```python
from build123d import *

# Parameters (mm, degrees)
SKETCH1_R           = 22.5
SKETCH1_R_2         = 15
SKETCH1_R_3         = 2
BOSS_EXTRUDE1_DEPTH = 5
SKETCH4_R           = 15
SKETCH4_R_2         = 10
SKETCH5_W           = 40
SKETCH5_H           = 40
SKETCH5_R           = 10
SKETCH5_R_2         = 2
BOSS_EXTRUDE2_DEPTH = 5
FILLET1_R           = 4
SKETCH6_R           = 3
BOSS_EXTRUDE3_DEPTH = 7


with BuildPart() as part:
    # Sketch1 → Boss-Extrude1 (new body)
    with BuildSketch(Plane.XY):
        Circle(SKETCH1_R)
        Circle(SKETCH1_R_2, mode=Mode.SUBTRACT)
        with Locations((13.177680547, 13.177680547)):
            Circle(SKETCH1_R_3, mode=Mode.SUBTRACT)
        with Locations((13.177680547, -13.177680547)):
            Circle(SKETCH1_R_3, mode=Mode.SUBTRACT)
        with Locations((-13.177680547, -13.177680547)):
            Circle(SKETCH1_R_3, mode=Mode.SUBTRACT)
        with Locations((-13.177680547, 13.177680547)):
            Circle(SKETCH1_R_3, mode=Mode.SUBTRACT)
    extrude(amount=BOSS_EXTRUDE1_DEPTH)

    # Sweep1: sweep along a path in Sketch3
    with BuildLine(Plane(origin=(0, 0, 0), x_dir=(1, 0, 0), z_dir=(0, 1, 0))) as sweep1_path:
        Line((0, 2.5), (0, -10))
        ThreePointArc((0, -10), (-11.757890636, -42.210884362), (-41.501642855, -59.272486499))
        Line((-41.501642855, -59.272486499), (-53.81976448, -61.397075786))
    # Sketch4 → Sweep1 (sweep)
    with BuildSketch(Plane(origin=(-53.81976448, 0, 61.397075786), x_dir=(0.16996714290024248, 0, 0.98544972998846), z_dir=(-0.98544972998846, 0, 0.16996714290024248))):
        Circle(SKETCH4_R)
        Circle(SKETCH4_R_2, mode=Mode.SUBTRACT)
    sweep(path=sweep1_path.line)

    # Sketch5 → Boss-Extrude2 (add)
    with BuildSketch(Plane(origin=(-62.548620892, 0, 10.788181337), x_dir=(0.16996714290024248, 0, 0.98544972998846), z_dir=(-0.98544972998846, 0, 0.16996714290024248))):
        with Locations((51.356140155, 0)):
            Rectangle(SKETCH5_W, SKETCH5_H)
        with Locations((51.356140155, 0)):
            Circle(SKETCH5_R, mode=Mode.SUBTRACT)
        with Locations((67.356140155, 16)):
            Circle(SKETCH5_R_2, mode=Mode.SUBTRACT)
        with Locations((35.356140155, 16)):
            Circle(SKETCH5_R_2, mode=Mode.SUBTRACT)
        with Locations((35.356140155, -16)):
            Circle(SKETCH5_R_2, mode=Mode.SUBTRACT)
        with Locations((67.356140155, -16)):
            Circle(SKETCH5_R_2, mode=Mode.SUBTRACT)
    extrude(amount=-BOSS_EXTRUDE2_DEPTH)

    # Fillet1
    fillet1_edges = [part.edges().sort_by_distance(p)[0] for p in [
        (-47.956797297, 20, 80.681152528),
        (-47.956797297, -20, 80.681152528),
        (-54.755483013, -20, 41.263163329),
        (-54.755483013, 20, 41.263163329),
    ]]
    fillet(fillet1_edges, radius=FILLET1_R)

    # Sketch6 → Boss-Extrude3 (add)
    with BuildSketch(Plane(origin=(0, -20, 0), x_dir=(-1, 0, 0), z_dir=(0, -1, 0))):
        with BuildLine():
            Line((48.89251583, -60.547240071), (47.830221187, -66.706300884))
            Line((47.830221187, -66.706300884), (42.902972537, -65.856465169))
            ThreePointArc((42.902972537, -65.856465169), (37.806206368, -58.635109714), (45.027561823, -53.538343544))
            Line((45.027561823, -53.538343544), (49.954810473, -54.388179259))
            Line((49.954810473, -54.388179259), (48.89251583, -60.547240071))
        make_face()
        with Locations(Location((43.96526718, -59.697404357, 0), (0, 0, 90))):
            Circle(SKETCH6_R, mode=Mode.SUBTRACT)
    extrude(amount=-BOSS_EXTRUDE3_DEPTH)


solid = part.part
```
CAD build for the part. Positions are in the model's coordinates, mm. A direction names the side the tool comes from. Give positions to 0.01 mm unless a question says otherwise; leave off trailing zeros. Order: outer loops, then holes, each group sorted by start corner. A loop starts at its lowest first (then second) coordinate and runs counter-clockwise, first axis right, second up.
(1) Tool access for faces 4 (the flat face through (15, -5, 0)), 5 (the flat face through (-47.43, 13.61, 69.03)), 6 (the flat face through (-45.401, -16.862, 66.287)), 7 (the flat face through (-51, 20, 61)): list every direction of +Z, -Z, +X, -X, +Y, -Y with a clear straight run to the whole face (end or side of a thin tool).
(2) Saw through at A-A, the plane y = -1. Give the cut face in (x, z).
(3) Saw through at C-C, the plane x = -21.5. State how many separate pieces and enclosed holes the cut face has, then the cut area to 3 significant figures.
(4) Drill centre lines: L1, parallel to Y at x = -13, z = 1; L2, parallel to X at y = 8, z = 42; L3, parallel to Z at x = -6, y = 17.5. Where is each one in solid material? Low to high.
(5) Flat gauge pins, fed straight in: pin 1 (1 mm diameter, centred on x = -1.5, z = 21, fed in from -Y); pin 2 (8 mm diameter, centred on x = -34, y = -10.5, fed in from +Z); pin 3 (6.5 mm diameter, centred on x = -13.18, y = -13.18, fed in from -Z). Where does each tip first touch, or does it go through?
(6) Saw through at B-B, the plane y = -5.5. Give the cut face in (x, z) (3 decimals), then the cut area to 3 significant figures.
(7) Mould opens along X. For faces 1 (the cylindrical face through (-2.17, -9.76, 3.84)), 2 (the cylindrical face through (-14.985, 0.66, -1.232)), 3 (the cylindrical face through (-54.527, 18.797, 42.381)) say: released by +X, released by -X, zero draft, split by the parting line, or undercut.
Results found:
1. face 4: -Z
1. face 5: none
1. face 6: +X, -Y
1. face 7: +Z, -Z, +X, -X, +Y
2. outline: (-57.22, 41.69) - (-52.29, 40.84) - (-51.44, 45.8) - (-44.05, 44.52) arc R35.03 cw to (-14.97, 10) - (-14.97, 5) - (-22.48, 5) - (-22.48, 0) - (-14.97, 0) - (-14.97, -2.5) - (-9.95, -2.5) - (-9.95, 10) arc R40.05 ccw to (-43.19, 49.47) - (-55.51, 51.59) - close; (-52.13, 71.2) - (-39.81, 69.08) arc R59.95 cw to (9.95, 10) - (9.95, -2.5) - (14.97, -2.5) - (14.97, 0) - (22.48, 0) - (22.48, 5) - (14.97, 5) - (14.97, 10) arc R64.97 ccw to (-38.96, 74.02) - (-46.35, 75.3) - (-45.49, 80.26) - (-50.42, 81.11) - close
3. separate pieces: 2
3. enclosed holes: 1
3. area: 566 mm2
4. L1: y = -18.36 to -15.17, -11.19 to 11.19, 15.17 to 18.36
4. L2: x = -57.17 to -52.09, -30.81 to -19.8, -4.04 to 3.91
4. L3: z = 0 to 5
5. pin 1: stops at y = -15
5. pin 2: stops at z = 71.69
5. pin 3: stops at z = 0
6. outline: (-57.219, 41.688) - (-52.292, 40.838) - (-51.264, 46.795) - (-43.874, 45.52) arc R36.045 cw to (-13.955, 10) - (-13.955, 5) - (-21.817, 5) - (-21.817, 0) - (-13.955, 0) - (-13.955, -2.5) - (-8.352, -2.5) - (-8.352, 10) arc R41.648 ccw to (-42.921, 51.042) - (-55.239, 53.167) - close; (-52.4, 69.627) - (-40.082, 67.503) arc R58.352 cw to (8.352, 10) - (8.352, -2.5) - (13.955, -2.5) - (13.955, 0) - (21.817, 0) - (21.817, 5) - (13.955, 5) - (13.955, 10) arc R63.955 ccw to (-39.13, 73.025) - (-46.521, 74.299) - (-45.493, 80.256) - (-50.42, 81.106) - close
6. area: 1,200 mm2
7. face 1: undercut
7. face 2: split by the parting line
7. face 3: released by -X
